Input: part model. Units: mm. Frame: model coordinates. Face numbers are marked on the shaded views. A direction names the side the tool comes from. Give positions to 0.01 mm unless a question says otherwise; leave off trailing zeros. Order: outer loops, then holes, each group sorted by start corner. A loop starts at its lowest first (then second) coordinate and runs counter-clockwise, first axis right, second up. Notation, with made-up numbers: M 3.25,63.25 L 32.25,63.25 A16 ccw 32.25,92.25 Z; hole C 89,19.25 d10. An arc over 180 degrees is marked long. Use a Markdown table: item, result.
from build123d import *

# Parameters (mm, degrees)
F1_DEPTH    = 33
F2_T        = 5
F2_T3_DEPTH = 43
F3_R        = 0.2
F4_R        = 0.5
F5_R        = 3
F6_R        = 1


# Not quite as in the source:
# - a shell that OpenCascade refuses in one call is made with other operations: the cavity is built on its own and cut out


with BuildPart() as f1:
    # F0 (on Right) → F1 (new body)
    with BuildSketch(Plane.YZ):
        Polygon((-20, 12), (-20, 0), (20, 0), (20, 12), (28, 12), (28, 63.5), (21, 63.5), (21, 52), (-21, 52), (-21, 63.5), (-28, 63.5), (-28, 12), align=None)
    extrude(amount=F1_DEPTH)

    # F2: shell of thickness 5, made by hand


with BuildPart() as f2_core1:
    # F2_t2: copy of F1
    add(f1.part)

    # the walls: a layer under each face that stays
    f2_faces = [f2_core1.faces().sort_by_distance(p)[0] for p in [
        (16.5, -20, 6),
        (16.5, 0, 0),
        (16.5, 20, 6),
        (16.5, 24, 12),
        (16.5, 28, 37.75),
        (16.5, 24.5, 63.5),
        (16.5, 21, 57.75),
        (16.5, 0, 52),
        (16.5, -21, 57.75),
        (16.5, -24.5, 63.5),
        (16.5, -28, 37.75),
        (16.5, -24, 12),
    ]]
    thicken(f2_faces, amount=-F2_T, mode=Mode.SUBTRACT)

    # F2_s4 → F2_t3 (cut)
    with BuildSketch(Plane.YZ.offset(-5)):
        Polygon((-20.05, 11.95), (-15, 12), (-15, 17), (-20, 17), align=None)
        Polygon((20.05, 11.95), (15, 12), (15, 17), (20, 17), align=None)
        Polygon((20.95, 52.05), (26, 52), (26, 47), (21, 47), align=None)
        Polygon((-20.95, 52.05), (-21, 47), (-26, 47), (-26, 52), align=None)
    extrude(amount=F2_T3_DEPTH, mode=Mode.SUBTRACT)


with BuildPart() as f1_1:
    add(f1.part)

    # what is left inside the walls is the cavity
    f2_cavity = [f2_core1.part.solids().sort_by_distance(p)[0] for p in [
        (32.95, 0, 19),
    ]]
    add(f2_cavity, mode=Mode.SUBTRACT)

    # F3
    f3_edges = [f1_1.edges().sort_by_distance(p)[0] for p in [
        (16.5, 20, 12),
        (16.5, -20, 12),
        (16.5, -21, 52),
        (16.5, 21, 52),
    ]]
    fillet(f3_edges, radius=F3_R)

    # F4
    f4_edges = [f1_1.edges().sort_by_distance(p)[0] for p in [
        (16.5, 21, 63.5),
        (16.5, 28, 63.5),
        (16.5, 28, 12),
        (16.5, 20, 0),
        (16.5, -20, 0),
        (16.5, -28, 12),
        (16.5, -28, 63.5),
        (16.5, -21, 63.5),
    ]]
    fillet(f4_edges, radius=F4_R)

    # F5
    f5_edges = [f1_1.edges().sort_by_distance(p)[0] for p in [
        (16.5, -23, 17),
        (16.5, 23, 17),
        (16.5, 15, 5),
        (16.5, -15, 5),
        (16.5, 23, 47),
        (16.5, -23, 47),
    ]]
    fillet(f5_edges, radius=F5_R)

    # F6
    f6_edges = [f1_1.edges().sort_by_distance(p)[0] for p in [
        (16.5, -15, 17),
        (16.5, 15, 17),
    ]]
    fillet(f6_edges, radius=F6_R)


solid = f1_1.part
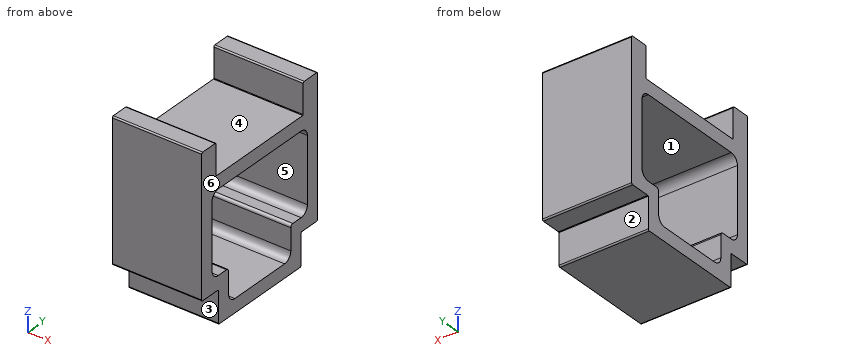
1) Cut plane B-B on y = 13.5. Return loops of the section in (x, z).
Response values:
| item | result |
|---|---|
| outline | M 0,0 L 33,0 L 33,5.4 L 0,5.4 Z; M 0,47 L 33,47 L 33,52 L 0,52 Z |
2) Cut plane A-A on z = 53.5. Return loops of the section in (x, y).
Response values:
| item | result |
|---|---|
| outline | M 0,-28 L 33,-28 L 33,-21 L 0,-21 Z; M 0,21 L 33,21 L 33,28 L 0,28 Z |
3) First-contact query: pin 1 Ø6 at (x, y) = (15, -24.5) entering from -Z; pin 2 Ø10 at (x, y) = (22.5, -6) entering from +Z; pin 3 Ø5.5 at (x, z) = (10, 5.5) entering from -Y. Flat tips, straight axial feed; report the tip coordinate or a pass-through.
Response values:
| item | result |
|---|---|
| pin 1 | stops at z = 12 |
| pin 2 | stops at z = 52 |
| pin 3 | stops at y = -20 |
4) Reachability of the marked faces 1, 2 and 3 from +Z, -Z, +X, -X, +Y, -Y: full face, straight path, thin tool, end or side. Return the list, or none.
Response values:
| item | result |
|---|---|
| face 1 | +X, -X |
| face 2 | -Z, +X, -X, +Y |
| face 3 | -Z, +X, -X, -Y |
5) Mould query, pull axis Z, two halves, no side actions, for the marked faces 4, 5 and 6. Classes: released by +Z, released by -Z, zero draft, split by the parting line, or undercut.
Response values:
| item | result |
|---|---|
| face 4 | released by +Z |
| face 5 | undercut |
| face 6 | zero draft |
6) Material intervals for line 1 (Z direction, x = 3, y = 3); line 2 (Y direction, x = 9, z = 42.5); line 3 (Y direction, x = 18, z = 60.5), sorted ascending. Write a range as from..to.
Response values:
| item | result |
|---|---|
| line 1 | z = 0..5, 47..52 |
| line 2 | y = -28..-23, 23..28 |
| line 3 | y = -28..-21, 21..28 |
